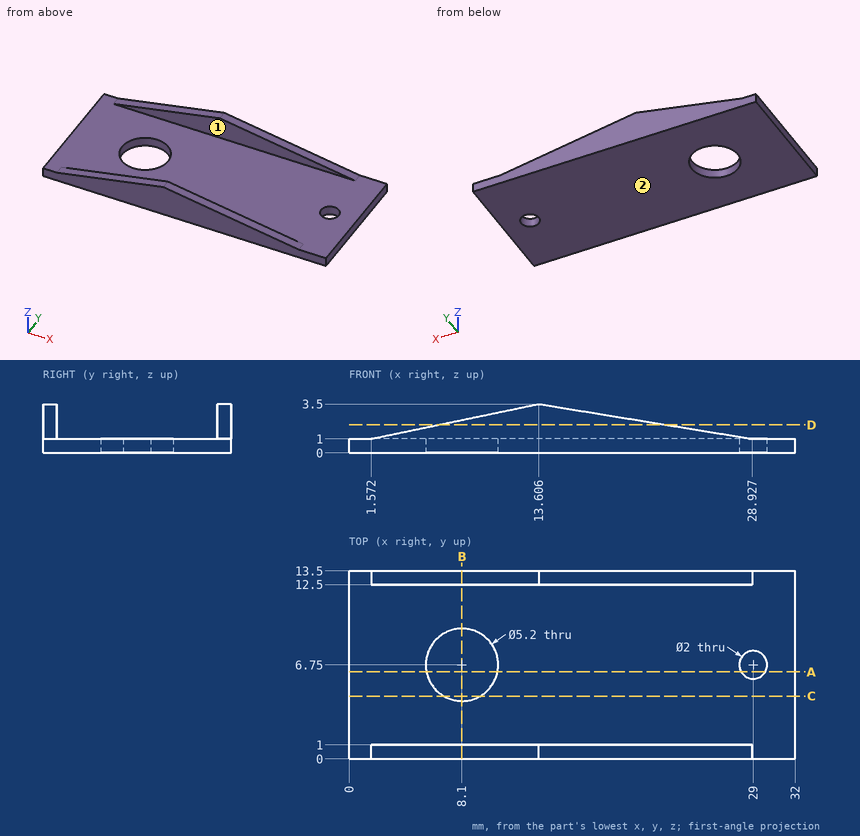
Design review of the part shown in the three views and the two pictorial views. Dimensions are in mm from the part's minimum x, y and z. A direction names the side the tool comes from. Round coordinates to 2 decimals unless told otherwise and drop trailing zeros. Order: outer loops, then holes, each group sorted by start corner. A loop starts at its lowest first (then second) coordinate and runs counter-clockwise, first axis right, second up. Notation, with made-up numbers: (63, 84.25) - (76, 84.25) arc R18 cw to (76, 98.25) - close; hole circle Ø11 at (-34, 11.5). An arc over 180 degrees is marked (long way). One line per question, with ' | ' between items.
Item 1: For P1, Ø4, axis at x = 8.5, y = 5.5, coming from the +Z side, flat-tipped, find the tip position at first contact; note if it passes through.
Checks:
P1: z = 1
Item 2: Take a section at D-D, the plane z = 2. Write out the cut boundary in (x, y) (1 decimal).
Checks:
outline: (6.4, 0) - (22.8, 0) - (22.8, 1) - (6.4, 1) - close; (6.4, 12.5) - (22.8, 12.5) - (22.8, 13.5) - (6.4, 13.5) - close
Item 3: Take a section at A-A, the plane y = 6.25. Write out the cut boundary in (x, z).
Checks:
outline: (0, 0) - (5.55, 0) - (5.55, 1) - (0, 1) - close; (10.65, 0) - (28.13, 0) - (28.13, 1) - (10.65, 1) - close; (29.87, 0) - (32, 0) - (32, 1) - (29.87, 1) - close
Item 4: Wall thickness on line 1 (Y direction, x = 8.1, z = 0.7); line 2 (Y direction, x = 29, z = 0.7); line 3 (Z direction, x = 4, y = 6.5): over which ranges is each line inside the solid? List them lowest first. Write a range as [from, to].
Checks:
line 1: [0, 4.15], [9.35, 13.5] | line 2: [0, 5.75], [7.75, 13.5] | line 3: [0, 1]
Item 5: Machinability: for the marked faces 1 and 2, which of the approach directions +Z, -Z, +X, -X, +Y, -Y give a long, thin tool a straight path to every point of the face, cutting with its end or side? Answer none if there is none.
Checks:
face 1: +Z, +X, -X | face 2: -Z, +X, -X, +Y, -Y
Item 6: Take a section at B-B, the plane x = 8.1. Write out the cut boundary in (y, z).
Checks:
outline: (0, 0) - (4.15, 0) - (4.15, 1) - (1, 1) - (1, 2.36) - (0, 2.36) - close; (9.35, 0) - (13.5, 0) - (13.5, 2.36) - (12.5, 2.36) - (12.5, 1) - (9.35, 1) - close
Item 7: Take a section at C-C, the plane y = 4.5. Write out the cut boundary in (x, z).
Checks:
outline: (0, 0) - (6.8, 0) - (6.8, 1) - (0, 1) - close; (9.4, 0) - (32, 0) - (32, 1) - (9.4, 1) - close
